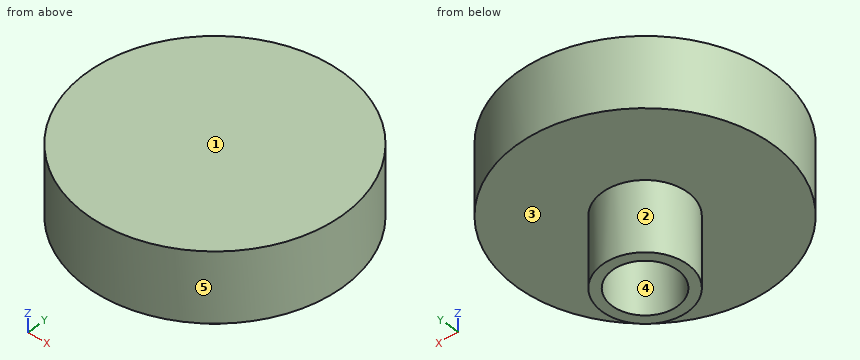
from build123d import *

# Parameters (mm, degrees)
F0_R     = 10.705893
F1_DEPTH = 5.842
F2_R     = 3.566194
F3_DEPTH = 5.842
F4_R     = 2.719536
F5_DEPTH = 5.5118
F6_R     = 2.717977
F7_DEPTH = 5.5118
F8_R     = 2.720478
F9_DEPTH = 5.5118


with BuildPart() as f1:
    # F0 (on Top) → F1 (new body)
    with BuildSketch(Plane.XY):
        Circle(F0_R)
    extrude(amount=F1_DEPTH)

    # F2 (on face) → F3 (join)
    with BuildSketch(Plane(origin=(0, 0, 0), x_dir=(1, 0, 0), z_dir=(0, 0, -1))):
        Circle(F2_R)
    extrude(amount=F3_DEPTH)

    # F4 (on face) → F5 (join)
    with BuildSketch(Plane(origin=(0, 0, -5.842), x_dir=(1, 0, 0), z_dir=(0, 0, -1))):
        Circle(F4_R)
    extrude(amount=-F5_DEPTH)

    # F6 (on face) → F7 (join)
    with BuildSketch(Plane(origin=(0, 0, -5.842), x_dir=(1, 0, 0), z_dir=(0, 0, -1))):
        Circle(F6_R)
    extrude(amount=-F7_DEPTH)

    # F8 (on face) → F9 (cut)
    with BuildSketch(Plane(origin=(0, 0, -5.842), x_dir=(1, 0, 0), z_dir=(0, 0, -1))):
        Circle(F8_R)
    extrude(amount=-F9_DEPTH, mode=Mode.SUBTRACT)


solid = f1.part
Geometry: final body of the model. Coordinates: model frame, mm. Face numbers are marked on the shaded views. A direction names the side the tool comes from. Coordinates: 2 decimals unless noted, no trailing zeros. Order: outer loops, then holes, each group sorted by start corner. A loop starts at its lowest first (then second) coordinate and runs counter-clockwise, first axis right, second up.
1) Set-up query: the marked faces 1 and 2. Return all of +Z, -Z, +X, -X, +Y, -Y with unobstructed straight access to the full face (end or side cutting, diameter ignored); none if empty.
Result sheet:
face 1: +Z, +X, -X, +Y, -Y
face 2: -Z
2) Section C-C (z = 1.25). Return loops of the section in (x, y).
Result sheet:
outline: circle Ø21.41 at (0, 0)
3) Draft query along Y for the marked faces 3, 4 and 5. Return one class per face: released by +Y, released by -Y, zero draft, split by the parting line, or undercut.
Result sheet:
face 3: zero draft
face 4: undercut
face 5: split by the parting line
4) Ray query, probe 1 along Y at (x, z) = (0, -4.45); probe 2 along Z at (x, y) = (-3, -9). Return the intervals inside material, ascending.
Result sheet:
probe 1: y = -3.57 to -2.72, 2.72 to 3.57
probe 2: z = 0 to 5.84
5) Section D-D (x = -4). Return loops of the section in (y, z), then the cut area to 3 significant figures.
Result sheet:
outline: (-9.93, 0) - (9.93, 0) - (9.93, 5.84) - (-9.93, 5.84) - close
area: 116 mm2
6) First-contact query: P1, Ø1.5, axis at y = 6, z = 2.5, coming from the +X side; P2, Ø6, axis at x = 5, z = 2, coming from the -Y side; P3, Ø1, axis at x = 6, y = 7, coming from the -Z side. Flat tips, straight axial feed; report the tip coordinate or a pass-through.
Result sheet:
P1: stops at x = 9.33
P2: stops at y = -10.52
P3: stops at z = 0
7) Section A-A (y = 0). Return loops of the section in (x, z).
Result sheet:
outline: (-10.71, 0) - (-3.57, 0) - (-3.57, -5.84) - (-2.72, -5.84) - (-2.72, -0.33) - (2.72, -0.33) - (2.72, -5.84) - (3.57, -5.84) - (3.57, 0) - (10.71, 0) - (10.71, 5.84) - (-10.71, 5.84) - close
